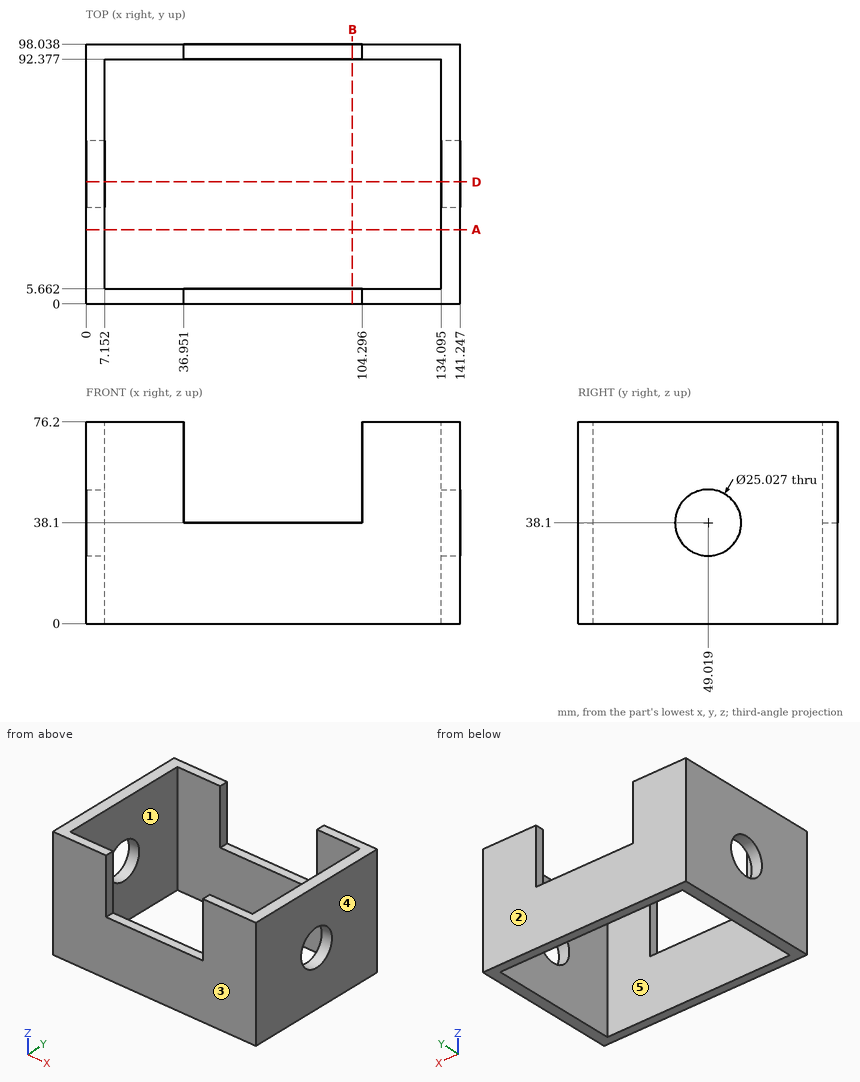
Here's the drawing with two shaded views (mm, measured from the low corner). I have some questions. A direction names the side the tool comes from. Give positions to 0.01 mm unless a question says otherwise; leave off trailing zeros. Order: outer loops, then holes, each group sorted by start corner. A loop starts at its lowest first (then second) coordinate and runs counter-clockwise, first axis right, second up.
Q1. Suppose I cut it at A-A, the plane y = 28. Write out the boundary of the cut face in (x, z) (1 decimal).
Q2. I'm going to push flat-ended pins straight in: P1, Ø15, axis at y = 49.02, z = 38.1, coming from the -X side; P2, Ø4.5, axis at x = 81.5, y = 94, coming from the +Z side. Where does each tip first touch, or does it pass through?
Q3. If I drill on line 1 along Y through (x, z) = (31.5, 52.5); line 2 along X through (y, z) = (55.5, 17.5) (1 decimal); line 3 along Z through (x, y) = (93, 5), over which ranges is the centre line in solid material (lowest first)?
Q4. For the marked faces 4 and 5, which set-ups out of +Z, -Z, +X, -X, +Y, -Y let a thin tool reach every point of the face, with its end or its side?
Q5. Suppose I cut it at B-B, the plane x = 100.5. Write out the boundary of the cut face in (y, z).
Q6. We'd pull the mould along Y, two halves only. Please class the marked faces 1, 2 and 3: +Y half, -Y half, draft (parallel to the pull), parting line (faces both ways), or undercut.
Q7. Suppose I cut it at D-D, the plane y = 46. Write out the boundary of the cut face in (x, z) (1 decimal).
Solution:
1. outline: (0, 0) - (7.2, 0) - (7.2, 76.2) - (0, 76.2) - close; (134.1, 0) - (141.2, 0) - (141.2, 76.2) - (134.1, 76.2) - close
2. P1: passes through
2. P2: stops at z = 38.1
3. line 1: y = 0 to 5.66, 92.38 to 98.04
3. line 2: x = 0 to 7.2, 134.1 to 141.2
3. line 3: z = 0 to 38.1
4. face 4: +Z, -Z, +X, +Y, -Y
4. face 5: +Z, -Z
5. outline: (0, 0) - (5.66, 0) - (5.66, 38.1) - (0, 38.1) - close; (92.38, 0) - (98.04, 0) - (98.04, 38.1) - (92.38, 38.1) - close
6. face 1: undercut
6. face 2: +Y half
6. face 3: -Y half
7. outline: (0, 0) - (7.2, 0) - (7.2, 26) - (0, 26) - close; (0, 50.2) - (7.2, 50.2) - (7.2, 76.2) - (0, 76.2) - close; (134.1, 0) - (141.2, 0) - (141.2, 26) - (134.1, 26) - close; (134.1, 50.2) - (141.2, 50.2) - (141.2, 76.2) - (134.1, 76.2) - close
